```python
from build123d import *

# Parameters (mm, degrees)
SKETCH1_R           = 4
BOSS_EXTRUDE1_DEPTH = 28


with BuildPart() as part:
    # Sketch1 → Boss-Extrude1 (new body)
    with BuildSketch(Plane(origin=(0, 0, 0), x_dir=(1, 0, 0), z_dir=(0, 1, 0))):
        with BuildLine():
            Line((76.845, -80.845), (76.845, -81.845))
            ThreePointArc((76.845, -81.845), (134.718154506, -57.873154506), (158.69, 0))
            ThreePointArc((158.69, 0), (153.69, 5), (148.69, 0))
            ThreePointArc((148.69, 0), (76.845, -71.845), (5, 0))
            ThreePointArc((5, 0), (-4.758823236, 1.534145171), (4.058559438, -2.920290275))
            ThreePointArc((4.058559438, -2.920290275), (78.305438675, -72.830358669), (149.69, 0))
            ThreePointArc((149.69, 0), (153.69, 4), (157.69, 0))
            ThreePointArc((157.69, 0), (134.011047725, -57.166047725), (76.845, -80.845))
        make_face()
        with Locations(Location((0, 0, 0), (0, 0, 270))):
            Circle(SKETCH1_R, mode=Mode.SUBTRACT)
    extrude(amount=BOSS_EXTRUDE1_DEPTH)


solid = part.part
```
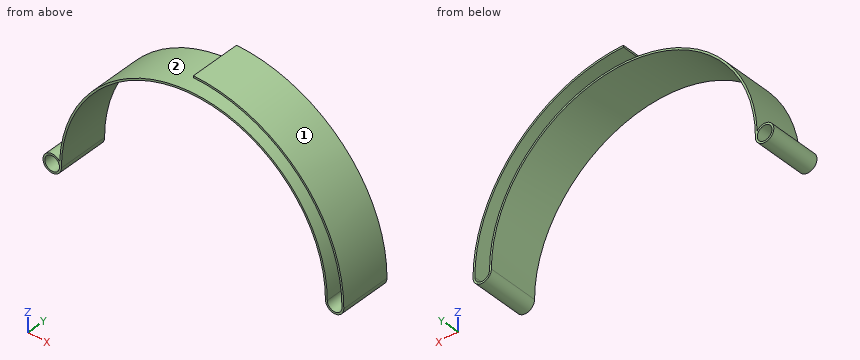
For this review, take the finished solid that the model builds, in its own axes (mm). Face numbers are marked on the shaded views. Coordinates: 2 decimals unless noted, no trailing zeros. Write each loop counter-clockwise with the first axis right and the second up, starting at its lowest first coordinate (ties: lowest second). Pieces come first, ordered by that corner, then holes. Notation, with made-up numbers: (81.5, -1.75) - (115.5, -1.75) arc R14 ccw to (115.5, 2.25) - close; hole circle Ø10 at (44, -22.5). An arc over 180 degrees is marked (long way). Put each result on its own line as item: value.
1. Add section D-D, the plane x = 144.5. Give the boundary of the cut face in (y, z), then the cut area to 3 significant figures.
Values found:
outline: (0, 24.18) - (28, 24.18) - (28, 27) - (0, 27) - close; (0, 44.26) - (28, 44.26) - (28, 46.06) - (0, 46.06) - close
area: 130 mm²
2. Wall thickness on probe 1 along X at (y, z) = (17.5, 42); probe 2 along X at (y, z) = (25, 66); probe 3 along X at (y, z) = (3.5, 1.5): over which ranges is each line inside the solid? List them lowest first.
Values found:
probe 1: 17.33 to 18.56, 135.13 to 136.36, 145.92 to 147.09
probe 2: 46.02 to 48.46, 105.23 to 107.67, 123.53 to 125.25
probe 3: -4.77 to -3.71, 3.71 to 5.02, 148.67 to 149.67, 157.68 to 158.68
3. For pin 1 (1 mm diameter, centred on x = 137.5, y = 7, fed in from +Z); pin 2 (3 mm diameter, centred on y = 22.5, z = 43, fed in from +X); pin 3 (2 mm diameter, centred on x = 40.5, y = 5, fed in from -Z); pin 4 (6.5 mm diameter, centred on x = 0, z = 0, fed in from -Y), all flat-tipped, find the tip position at first contact; note any pin that passes through.
Values found:
pin 1: z = 55.5
pin 2: x = 147.39
pin 3: z = 61.38
pin 4: through
4. Add section C-C, the plane y = 12.5. Give the boundary of the cut face in (x, z) (3 decimals).
Values found:
outline: (4.059, 2.92) arc R5 ccw (long way) to (5, 0) arc R71.845 cw to (148.69, 0) arc R5 ccw to (158.69, 0) arc R81.845 ccw to (76.845, 81.845) - (76.845, 80.845) arc R80.845 cw to (157.69, 0) arc R4 cw to (149.69, 0) arc R72.845 ccw to start; hole circle Ø8 at (0, 0)
5. Add section A-A, the plane x = 0. Give the boundary of the cut face in (y, z), then the cut area to 3 significant figures.
Values found:
outline: (0, -5) - (28, -5) - (28, -4) - (0, -4) - close; (0, 4) - (28, 4) - (28, 5) - (0, 5) - close
area: 56.0 mm²
6. Mouldability with a two-part tool opening along X and no side actions: class the marked faces 1 and 2 as released by +X, released by -X, zero draft, split by the parting line, or undercut.
Values found:
face 1: released by +X
face 2: undercut
